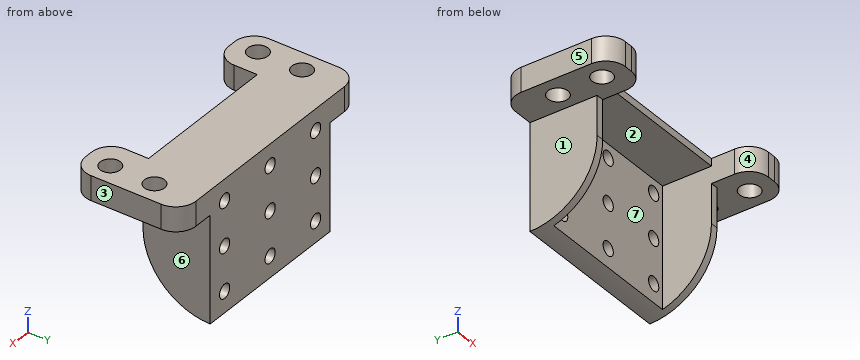
from build123d import *

# Parameters (mm, degrees)
F0_W          = 27
F0_H          = 21.4
F1_DEPTH      = 3
F2_R          = 1.15
F3_DEPTH      = 3.001
F5_DEPTH      = 8
F5_DEPTH_BACK = 3
F6_W          = 7.75
F6_H          = 4
F7_DEPTH      = 7
F8_R          = 1.65
F9_DEPTH      = 25
F10_F1_R      = 10.9999
F11_R         = 3.3
F12_R         = 3.2


# Not quite as in the source:
# - a fillet or chamfer is up to 0.001 mm smaller than in the source, because OpenCascade refuses the exact size


with BuildPart() as f1:
    # F0 (on Front) → F1 (new body)
    with BuildSketch(Plane.XZ):
        Rectangle(F0_W, F0_H)
    extrude(amount=-F1_DEPTH)

    # F2 (on Front) → F3 (cut, through all)
    with BuildSketch(Plane.XZ):
        with Locations((0, 7.225)):
            Circle(F2_R)
        Circle(F2_R)
        with Locations((0, -7.225)):
            Circle(F2_R)
        with Locations((10.25, 0)):
            Circle(F2_R)
        with Locations((10.25, 7.225)):
            Circle(F2_R)
        with Locations((10.25, -7.225)):
            Circle(F2_R)
        with Locations((-10.25, -7.225)):
            Circle(F2_R)
        with Locations((-10.25, 0)):
            Circle(F2_R)
        with Locations((-10.25, 7.225)):
            Circle(F2_R)
    extrude(amount=-F3_DEPTH, mode=Mode.SUBTRACT)

    # F4 (on Front) → F5 (join, two sides)
    with BuildSketch(Plane.XZ) as f5_sk:
        Polygon((20, 10.7), (0, 10.7), (-20, 10.7), (-20, 6.7), (-13.5, 6.7), (-13.5, -10.7), (-12.25, -10.7), (-12.25, 9.475), (0, 9.475), (12.25, 9.475), (12.25, -10.7), (13.5, -10.7), (13.5, 6.7), (20, 6.7), align=None)
    extrude(amount=F5_DEPTH)
    extrude(f5_sk.sketch, amount=-F5_DEPTH_BACK)

    # F6 (on face) → F7 (join)
    with BuildSketch(Plane.XZ.offset(8)):
        with Locations((16.125, 8.7)):
            Rectangle(F6_W, F6_H)
        with Locations((-16.125, 8.7)):
            Rectangle(F6_W, F6_H)
    extrude(amount=F7_DEPTH)

    # F8 (on face) → F9 (cut)
    with BuildSketch(Plane(origin=(0, 0, 6.7), x_dir=(1, 0, 0), z_dir=(0, 0, -1))):
        with Locations((-16.625, 3.85)):
            Circle(F8_R)
        with Locations((16.625, 3.85)):
            Circle(F8_R)
        with Locations((16.625, 11.075)):
            Circle(F8_R)
        with Locations((-16.625, 11.075)):
            Circle(F8_R)
    extrude(amount=-F9_DEPTH, mode=Mode.SUBTRACT)

    # F10: fillet of radius 11 on 2 edges, made by hand

    # F10_f1 (radius 11 in the source; OpenCascade refuses exactly that, so slightly less here)
    f10_f1_edges = [f1.edges().sort_by_distance(p)[0] for p in [
        (12.875, -8, -10.7),
    ]]
    fillet(f10_f1_edges, radius=F10_F1_R)

    # F11
    f11_edges = [f1.edges().sort_by_distance(p)[0] for p in [
        (20, 3, 8.7),
        (-20, 3, 8.7),
    ]]
    fillet(f11_edges, radius=F11_R)

    # F12
    f12_edges = [f1.edges().sort_by_distance(p)[0] for p in [
        (20, -15, 8.7),
        (12.25, -15, 8.7),
        (-12.25, -15, 8.7),
        (-20, -15, 8.7),
    ]]
    fillet(f12_edges, radius=F12_R)


solid = f1.part
Geometry check sheet. Reference: the model listing, model coordinates, mm. Face numbers are marked on the shaded views. A direction names the side the tool comes from. Coordinates: 2 decimals unless noted, no trailing zeros. Order: outer loops, then holes, each group sorted by start corner. A loop starts at its lowest first (then second) coordinate and runs counter-clockwise, first axis right, second up. Notation, with made-up numbers: (31.5, -31) - (77.5, -31) arc R24 cw to (77.5, -10) - close; hole circle Ø9 at (-37, 20). An arc over 180 degrees is marked (long way). Answer in a Markdown table with one row per item. Add a question column.
1) Release check for a two-part mould opening along X. For the marked faces 1, 2 and 3 record: +X half, -X half, draft (parallel to the pull), parting line (faces both ways), or undercut.
2) Material ranges on line 1 along X through (y, z) = (-3.85, 7.9) (3 decimals); line 2 along X through (y, z) = (-3.5, 5.25); line 3 along Z through (x, y) = (-10.25, 1.5) (3 decimals), recorded low to high. Write a range as [from, to].
3) Cross-section at B-B, the plane y = -2.75. Record the cut outline in (x, z) (3 decimals), then the cut area to 3 significant figures.
4) Set-up check for the marked faces 4, 5, 6 and 7: record each of +Z, -Z, +X, -X, +Y, -Y from which the full face is reachable in a straight line by a thin tool's end or side.
5) Cross-section at C-C, the plane y = -10. Record the cut outline in (x, z), then the cut area to 3 significant figures.
6) Cross-section at A-A, the plane x = 0. State how many separate pieces and enclosed holes the cut face has, then the cut area to 3 significant figures.
7) Cross-section at D-D, the plane z = 3. Record the cut outline in (x, y).
8) Gauge pin test, flat ends, axial feed: P1, Ø1.4, axis at x = -10.25, z = 7.225, coming from the -Y side; P2, Ø4.5, axis at x = 16.625, y = -3.85, coming from the -Z side; P3, Ø1.5, axis at y = -1, z = -3, coming from the +X side; P4, Ø2, axis at x = 14, z = -0.5, coming from the -Y side. Record the tip position at first contact, or that the pin passes through.
Check result:
| question | item | result |
|---|---|---|
| 1 | face 1 | -X half |
| 1 | face 2 | undercut |
| 1 | face 3 | +X half |
| 2 | line 1 | x = [-20, -18.275], [-14.975, -12.25], [12.25, 14.975], [18.275, 20] |
| 2 | line 2 | x = [-13.5, -12.25], [12.25, 13.5] |
| 2 | line 3 | z = [-10.597, -8.375], [-6.075, -1.15], [1.15, 6.075], [8.375, 10.7] |
| 3 | outline | (-20, 6.7) - (-17.855, 6.7) - (-17.855, 10.7) - (-20, 10.7) - close; (-15.395, 6.7) - (-13.5, 6.7) - (-13.5, -9.078) - (-12.25, -9.078) - (-12.25, 9.475) - (12.25, 9.475) - (12.25, -9.078) - (13.5, -9.078) - (13.5, 6.7) - (15.395, 6.7) - (15.395, 10.7) - (-15.395, 10.7) - close; (17.855, 6.7) - (20, 6.7) - (20, 10.7) - (17.855, 10.7) - close |
| 3 | area | 112 mm² |
| 4 | face 4 | +Z, -Z, -Y |
| 4 | face 5 | +Z, -Z, -X, +Y, -Y |
| 4 | face 6 | -Z, +X, +Y, -Y |
| 4 | face 7 | -Z, -Y |
| 5 | outline | (-20, 6.7) - (-17.88, 6.7) - (-17.88, 10.7) - (-20, 10.7) - close; (-15.37, 6.7) - (-12.25, 6.7) - (-12.25, 10.7) - (-15.37, 10.7) - close; (12.25, 6.7) - (15.37, 6.7) - (15.37, 10.7) - (12.25, 10.7) - close; (17.88, 6.7) - (20, 6.7) - (20, 10.7) - (17.88, 10.7) - close |
| 5 | area | 42.0 mm² |
| 6 | separate pieces | 4 |
| 6 | enclosed holes | 0 |
| 6 | area | 52.9 mm² |
| 7 | outline | (-13.5, -8) - (-12.25, -8) - (-12.25, 0) - (12.25, 0) - (12.25, -8) - (13.5, -8) - (13.5, 3) - (-13.5, 3) - close |
| 8 | P1 | passes through |
| 8 | P2 | stops at z = 6.7 |
| 8 | P3 | stops at x = 13.5 |
| 8 | P4 | stops at y = -8 |
